```python
from build123d import *

# Parameters (mm, degrees)
F1_DEPTH = 3
F2_DEPTH = 2.5
F3_DEPTH = 2
F4_DEPTH = 1.5
F5_DEPTH = 1


with BuildPart() as f1:
    # F0 (on Top) → F1 (new body)
    with BuildSketch(Plane.XY):
        with BuildLine():
            ThreePointArc((0, 2.5), (-1.767766953, 1.767766953), (-2.5, 0))
            ThreePointArc((-2.5, 0), (-1.767766953, -1.767766953), (0, -2.5))
            ThreePointArc((0, -2.5), (1.767766953, -1.767766953), (2.5, 0))
            ThreePointArc((2.5, 0), (1.767766953, 1.767766953), (0, 2.5))
        make_face()
        with BuildLine():
            Line((-2.5, 0), (-2.5, 14.7901994577))
            ThreePointArc((-2.5, 14.7901994577), (-12.2260172846, 8.6904833787), (-14.7901994577, -2.5))
            Line((-14.7901994577, -2.5), (-3.8416876048, -2.5))
            ThreePointArc((-3.8416876048, -2.5), (-2.8566179631, -1.4186371655), (-2.5, 0))
        make_face()
        with BuildLine():
            Line((3.8416876048, 2.5), (14.7901994577, 2.5))
            ThreePointArc((14.7901994577, 2.5), (8.6904833787, 12.2260172846), (-2.5, 14.7901994577))
            Line((-2.5, 14.7901994577), (-2.5, 0))
            ThreePointArc((-2.5, 0), (-1.767766953, 1.767766953), (0, 2.5))
            Line((0, 2.5), (3.8416876048, 2.5))
        make_face()
        with BuildLine():
            ThreePointArc((2.5, 0), (2.8566179631, 1.4186371655), (3.8416876048, 2.5))
            Line((3.8416876048, 2.5), (0, 2.5))
            ThreePointArc((0, 2.5), (1.767766953, 1.767766953), (2.5, 0))
        make_face()
        with BuildLine():
            ThreePointArc((2.5, -14.7901994577), (11.4564392374, -9.6824583655), (15, 0))
            ThreePointArc((15, 0), (14.9474578418, 1.2543939042), (14.7901994577, 2.5))
            Line((14.7901994577, 2.5), (3.8416876048, 2.5))
            ThreePointArc((3.8416876048, 2.5), (2.8566179631, 1.4186371655), (2.5, 0))
            Line((2.5, 0), (2.5, -3.8416876048))
            Line((2.5, -3.8416876048), (2.5, -14.7901994577))
        make_face()
        with BuildLine():
            ThreePointArc((0, -2.5), (1.4186371655, -2.8566179631), (2.5, -3.8416876048))
            Line((2.5, -3.8416876048), (2.5, 0))
            ThreePointArc((2.5, 0), (1.767766953, -1.767766953), (0, -2.5))
        make_face()
        with BuildLine():
            ThreePointArc((-14.7901994577, -2.5), (-8.6904833787, -12.2260172846), (2.5, -14.7901994577))
            Line((2.5, -14.7901994577), (2.5, -3.8416876048))
            ThreePointArc((2.5, -3.8416876048), (1.4186371655, -2.8566179631), (0, -2.5))
            Line((0, -2.5), (-3.8416876048, -2.5))
            Line((-3.8416876048, -2.5), (-14.7901994577, -2.5))
        make_face()
        with BuildLine():
            ThreePointArc((0, -2.5), (-1.767766953, -1.767766953), (-2.5, 0))
            ThreePointArc((-2.5, 0), (-2.8566179631, -1.4186371655), (-3.8416876048, -2.5))
            Line((-3.8416876048, -2.5), (0, -2.5))
        make_face()
    extrude(amount=F1_DEPTH)

    # F0 (on Top) → F2 (cut)
    with BuildSketch(Plane.XY):
        with BuildLine():
            Line((-2.5, 0), (-2.5, 14.7901994577))
            ThreePointArc((-2.5, 14.7901994577), (-12.2260172846, 8.6904833787), (-14.7901994577, -2.5))
            Line((-14.7901994577, -2.5), (-3.8416876048, -2.5))
            ThreePointArc((-3.8416876048, -2.5), (-2.8566179631, -1.4186371655), (-2.5, 0))
        make_face()
    extrude(amount=F2_DEPTH, mode=Mode.SUBTRACT)

    # F0 (on Top) → F3 (cut)
    with BuildSketch(Plane.XY):
        with BuildLine():
            ThreePointArc((-14.7901994577, -2.5), (-8.6904833787, -12.2260172846), (2.5, -14.7901994577))
            Line((2.5, -14.7901994577), (2.5, -3.8416876048))
            ThreePointArc((2.5, -3.8416876048), (1.4186371655, -2.8566179631), (0, -2.5))
            Line((0, -2.5), (-3.8416876048, -2.5))
            Line((-3.8416876048, -2.5), (-14.7901994577, -2.5))
        make_face()
        with BuildLine():
            ThreePointArc((0, -2.5), (-1.767766953, -1.767766953), (-2.5, 0))
            ThreePointArc((-2.5, 0), (-2.8566179631, -1.4186371655), (-3.8416876048, -2.5))
            Line((-3.8416876048, -2.5), (0, -2.5))
        make_face()
    extrude(amount=F3_DEPTH, mode=Mode.SUBTRACT)

    # F0 (on Top) → F4 (cut)
    with BuildSketch(Plane.XY):
        with BuildLine():
            ThreePointArc((2.5, -14.7901994577), (11.4564392374, -9.6824583655), (15, 0))
            ThreePointArc((15, 0), (14.9474578418, 1.2543939042), (14.7901994577, 2.5))
            Line((14.7901994577, 2.5), (3.8416876048, 2.5))
            ThreePointArc((3.8416876048, 2.5), (2.8566179631, 1.4186371655), (2.5, 0))
            Line((2.5, 0), (2.5, -3.8416876048))
            Line((2.5, -3.8416876048), (2.5, -14.7901994577))
        make_face()
        with BuildLine():
            ThreePointArc((0, -2.5), (1.4186371655, -2.8566179631), (2.5, -3.8416876048))
            Line((2.5, -3.8416876048), (2.5, 0))
            ThreePointArc((2.5, 0), (1.767766953, -1.767766953), (0, -2.5))
        make_face()
    extrude(amount=F4_DEPTH, mode=Mode.SUBTRACT)

    # F0 (on Top) → F5 (cut)
    with BuildSketch(Plane.XY):
        with BuildLine():
            Line((3.8416876048, 2.5), (14.7901994577, 2.5))
            ThreePointArc((14.7901994577, 2.5), (8.6904833787, 12.2260172846), (-2.5, 14.7901994577))
            Line((-2.5, 14.7901994577), (-2.5, 0))
            ThreePointArc((-2.5, 0), (-1.767766953, 1.767766953), (0, 2.5))
            Line((0, 2.5), (3.8416876048, 2.5))
        make_face()
        with BuildLine():
            ThreePointArc((2.5, 0), (2.8566179631, 1.4186371655), (3.8416876048, 2.5))
            Line((3.8416876048, 2.5), (0, 2.5))
            ThreePointArc((0, 2.5), (1.767766953, 1.767766953), (2.5, 0))
        make_face()
    extrude(amount=F5_DEPTH, mode=Mode.SUBTRACT)


solid = f1.part
```
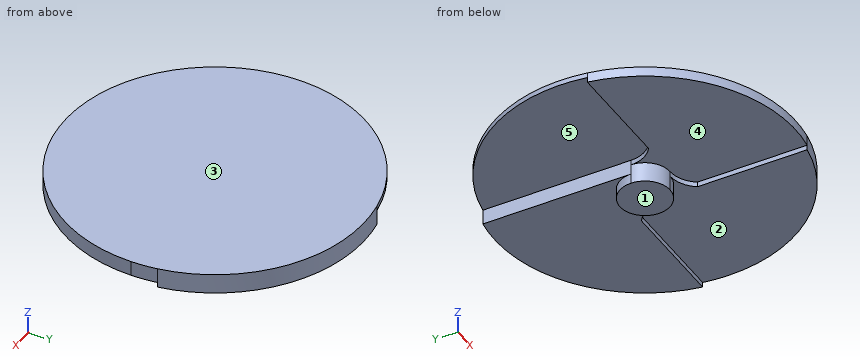
Design review of the part built by this model. Coordinates are the model's own, in mm. Face numbers are marked on the shaded views. A direction names the side the tool comes from. Round coordinates to 2 decimals unless told otherwise and drop trailing zeros. Write each loop counter-clockwise with the first axis right and the second up, starting at its lowest first coordinate (ties: lowest second). Pieces come first, ordered by that corner, then holes. Notation, with made-up numbers: (-2, 11.5) -> (56, 11.5) arc R9 ccw to (56, 26.5) -> close; hole circle Ø7 at (68, 58). An arc over 180 degrees is marked (long way). Write item = value, one per line. Start each with the question number.
1) Take a section at A-A, the plane y = -0.75. State the section outline as (x, z) points, plus the area to 3 significant figures.
2) Clearance check with flat-ended pins moving along their axes: pin 1 (1 mm diameter, centred on x = 7.5, y = -2.5, fed in from -Z); pin 2 (1 mm diameter, centred on x = -10, y = -7.5, fed in from -Z); pin 3 (7.5 mm diameter, centred on x = 5.5, y = 4, fed in from -Z). State where each tip first meets the part, or that it passes through.
3) Tool access review of the marked faces 1, 2, 3, 4 and 5: name each direction out of +Z, -Z, +X, -X, +Y, -Y from which nothing blocks a thin tool from reaching the whole face with its end or side.
4) Wall thickness on probe 1 along Z at (x, y) = (2, -2.5); probe 2 along Z at (x, y) = (8, 7.25); probe 3 along X at (y, z) = (-2.25, 0.6): over which ranges is each line inside the solid? List them lowest first. Write a range as from..to.
5) Take a section at D-D, the plane y = -4.75. State the section outline as (x, z) points.
6) Take a section at C-C, the plane x = -5. State the section outline as (y, z) points.
7) Take a section at B-B, the plane z = 0.45. State the section outline as (x, y) points, plus the area to 3 significant figures.
Results list:
q1.outline = (-14.98, 2.5) -> (-2.6, 2.5) -> (-2.6, 2) -> (-2.38, 2) -> (-2.38, 0) -> (2.38, 0) -> (2.38, 1.5) -> (14.98, 1.5) -> (14.98, 3) -> (-14.98, 3) -> close
q1.area = 39.6 mm²
q2.pin_1 = 1.5
q2.pin_2 = 2
q2.pin_3 = 1
q3.face_1 = -Z, +X, -X, +Y, -Y
q3.face_2 = -Z, +X, -Y
q3.face_3 = +Z, +X, -X, +Y, -Y
q3.face_4 = -Z, -X, -Y
q3.face_5 = -Z, -X, +Y
q4.probe_1 = 1.5..3
q4.probe_2 = 1..3
q4.probe_3 = -1.09..1.09
q5.outline = (-14.23, 2) -> (2.5, 2) -> (2.5, 1.5) -> (14.23, 1.5) -> (14.23, 3) -> (-14.23, 3) -> close
q6.outline = (-14.14, 2) -> (-2.5, 2) -> (-2.5, 2.5) -> (14.14, 2.5) -> (14.14, 3) -> (-14.14, 3) -> close
q7.outline = circle Ø5 at (0, 0)
q7.area = 19.6 mm²
